Source: CAD feature listing. Evaluate the final solid. Frame: model axes, mm. A direction names the side the tool comes from. Round coordinates to 2 decimals unless told otherwise and drop trailing zeros. Order: outer loops, then holes, each group sorted by start corner. A loop starts at its lowest first (then second) coordinate and runs counter-clockwise, first axis right, second up. Notation, with made-up numbers: (51.5, -37) - (68.5, -37) arc R3 cw to (68.5, -33) - close; hole circle Ø11 at (69.5, 11.25). An arc over 180 degrees is marked (long way). Put each result on its own line as item: value. Start each with the question number.
1) Access query for faces 4 (the face through (12.066, 12.099, -3620.389)), 5 (the face through (11.176, 0, -3620)). Directions: +Z, -Z, +X, -X, +Y, -Y. A direction counts if a zero-diameter tool reaches every point of the face in a straight line with its end or side. Return the directions, or none.
2) Section A-A on y = -7.25. Output: boundary loops of the cut face in (x, z).
3) Line query: probe 1 along X at (y, z) = (-0.75, -3602); probe 2 along X at (y, z) = (11.5, -3607.5). Output: solid intervals per line, ascending. Write a range as [from, to].
4) Mould query, pull axis Y, two halves, no side actions, for faces 1 (the face through (0, -11.176, -3620)), 2 (the face through (12.7, 0, -3620)), 3 (the face through (0, -12.7, -3620)). Classes: +Y half, -Y half, draft (parallel to the pull), parting line (faces both ways), or undercut.
5) Section C-C on z = -3599. Output: boundary loops of the cut face in (x, y), then the cut area to 3 significant figures.
6) Contact query for a flat-ended pin moving along its axis: P1, Ø10, axis at x = 0, y = 3.5, coming from the -Z side. Output: stop coordinate, or through.
```python
from build123d import *

# Parameters (mm, degrees)
BOSS_EXTRUDE1_DEPTH = 127


with BuildPart() as part:
    # Sketch1 → Boss-Extrude1 (new body)
    with BuildSketch(Plane(origin=(0, 0, -3683), x_dir=(-1, 0, 0), z_dir=(0, 0, -1))):
        with BuildLine():
            Line((12.7, -10.5918), (12.7, 10.5918))
            ThreePointArc((12.7, 10.5918), (12.082522516, 12.082522516), (10.5918, 12.7))
            Line((10.5918, 12.7), (-10.5918, 12.7))
            ThreePointArc((-10.5918, 12.7), (-12.082522516, 12.082522516), (-12.7, 10.5918))
            Line((-12.7, 10.5918), (-12.7, -10.5918))
            ThreePointArc((-12.7, -10.5918), (-12.082522516, -12.082522516), (-10.5918, -12.7))
            Line((-10.5918, -12.7), (10.5918, -12.7))
            ThreePointArc((10.5918, -12.7), (12.082522516, -12.082522516), (12.7, -10.5918))
        make_face()
        with BuildLine():
            Line((11.176, 9.652), (11.176, -9.652))
            ThreePointArc((11.176, -9.652), (10.729630735, -10.729630735), (9.652, -11.176))
            Line((9.652, -11.176), (-9.652, -11.176))
            ThreePointArc((-9.652, -11.176), (-10.729630735, -10.729630735), (-11.176, -9.652))
            Line((-11.176, -9.652), (-11.176, 9.652))
            ThreePointArc((-11.176, 9.652), (-10.729630735, 10.729630735), (-9.652, 11.176))
            Line((-9.652, 11.176), (9.652, 11.176))
            ThreePointArc((9.652, 11.176), (10.729630735, 10.729630735), (11.176, 9.652))
        make_face(mode=Mode.SUBTRACT)
    extrude(amount=-BOSS_EXTRUDE1_DEPTH)


solid = part.part
```
Answer sheet:
1. face 4: +Z, -Z, +X, +Y
1. face 5: +Z, -Z
2. outline: (-12.7, -3683) - (-11.18, -3683) - (-11.18, -3556) - (-12.7, -3556) - close; (11.18, -3683) - (12.7, -3683) - (12.7, -3556) - (11.18, -3556) - close
3. probe 1: [-12.7, -11.18], [11.18, 12.7]
3. probe 2: [-12.49, 12.49]
4. face 1: undercut
4. face 2: draft
4. face 3: -Y half
5. outline: (-12.7, -10.59) arc R2.11 ccw to (-10.59, -12.7) - (10.59, -12.7) arc R2.11 ccw to (12.7, -10.59) - (12.7, 10.59) arc R2.11 ccw to (10.59, 12.7) - (-10.59, 12.7) arc R2.11 ccw to (-12.7, 10.59) - close; hole (-11.18, -9.65) arc R1.52 ccw to (-9.65, -11.18) - (9.65, -11.18) arc R1.52 ccw to (11.18, -9.65) - (11.18, 9.65) arc R1.52 ccw to (9.65, 11.18) - (-9.65, 11.18) arc R1.52 ccw to (-11.18, 9.65) - close
5. area: 144 mm^2
6. P1: through
